The model under review builds one solid part; all positions refer to its coordinate system, in mm. Face numbers are marked on the shaded views. A direction names the side the tool comes from. Round coordinates to 2 decimals unless told otherwise and drop trailing zeros. Order: outer loops, then holes, each group sorted by start corner. A loop starts at its lowest first (then second) coordinate and runs counter-clockwise, first axis right, second up. Notation, with made-up numbers: M 74,18 L 94,18 A20 cw 94,23 Z; hole C 57,13 d10. An arc over 180 degrees is marked long. Answer as a JSON object with one key per item and string values. Group by question number.
1. Clearance check with flat-ended pins moving along their axes: P1, Ø12.5, axis at x = 15.5, y = 56.5, coming from the +Z side; P2, Ø1.5, axis at x = 30.5, z = 59.5, coming from the +Y side; P3, Ø6, axis at x = 25, y = 54, coming from the +Z side. State where each tip first meets the part, or that it passes through.
2. Add section C-C on z = 29.5. State the section outline as (x, y) points, and give its area (3 significant figures).
3. To check wall thickness, follow probe 1 along Y at (x, z) = (46.5, 38.5); probe 2 along Z at (x, y) = (35, 51.5); probe 3 along Z at (x, y) = (24, 72). State the ranges of each line that lie inside material, in increasing order. Write a range as [from, to].
4. Machinability: for the marked faces 1, 2 and 3, which of the approach directions +Z, -Z, +X, -X, +Y, -Y give a long, thin tool a straight path to every point of the face, cutting with its end or side? Answer none if there is none.
```python
from build123d import *

# Parameters (mm, degrees)
F1_DEPTH = 25.4
F2_W     = 25.4
F2_H     = 25.4
F3_DEPTH = 50.8
F4_R     = 25.39999


# Not quite as in the source:
# - a fillet or chamfer is up to 0.001 mm smaller than in the source, because OpenCascade refuses the exact size


with BuildPart() as f1:
    # F0 (on Top) → F1 (new body)
    with BuildSketch(Plane.XY):
        Polygon((0, 76.2), (0, 0), (25.4, 0), (25.4, 50.8), (50.8, 50.8), (50.8, 76.2), align=None)
    extrude(amount=F1_DEPTH)

    # F2 (on face) → F3 (join)
    with BuildSketch(Plane.XY.offset(25.4)):
        with Locations((38.1, 63.5)):
            Rectangle(F2_W, F2_H)
    extrude(amount=F3_DEPTH)

    # F4 (radius 25.4 in the source; OpenCascade refuses exactly that, so slightly less here)
    f4_edges = [f1.edges().sort_by_distance(p)[0] for p in [
        (0, 38.1, 0),
        (0, 0, 12.7),
        (0, 76.2, 12.7),
        (25.4, 76.2, 0),
        (38.1, 76.2, 76.2),
        (12.7, 0, 0),
    ]]
    fillet(f4_edges, radius=F4_R)


solid = f1.part
```
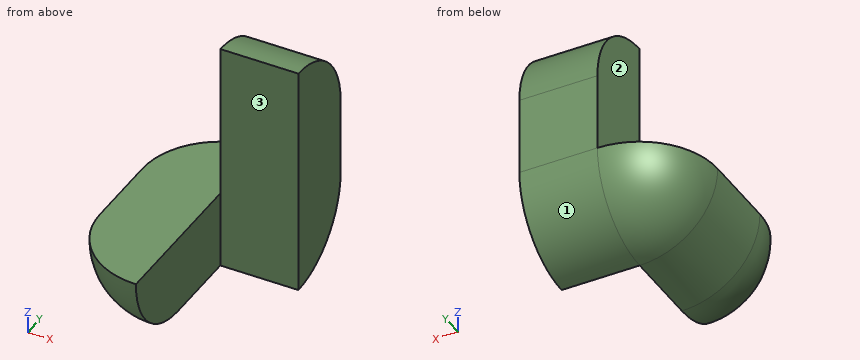
Recorded:
{
 "1": {"P1": "stops at z = 25.4", "P2": "stops at y = 74.92", "P3": "stops at z = 76.2"},
 "2": {"outline": "M 25.4,50.8 L 50.8,50.8 L 50.8,76.2 L 25.4,76.2 Z", "area": "645 mm²"},
 "3": {"probe 1": "y = [50.8, 76.2]", "probe 2": "z = [0.01, 76.19]", "probe 3": "z = [11.48, 25.4]"},
 "4": {"face 1": "-Z, +X, -X, +Y", "face 2": "+Z, -X, +Y, -Y", "face 3": "+Z, -Z, +X, -Y"}
}
